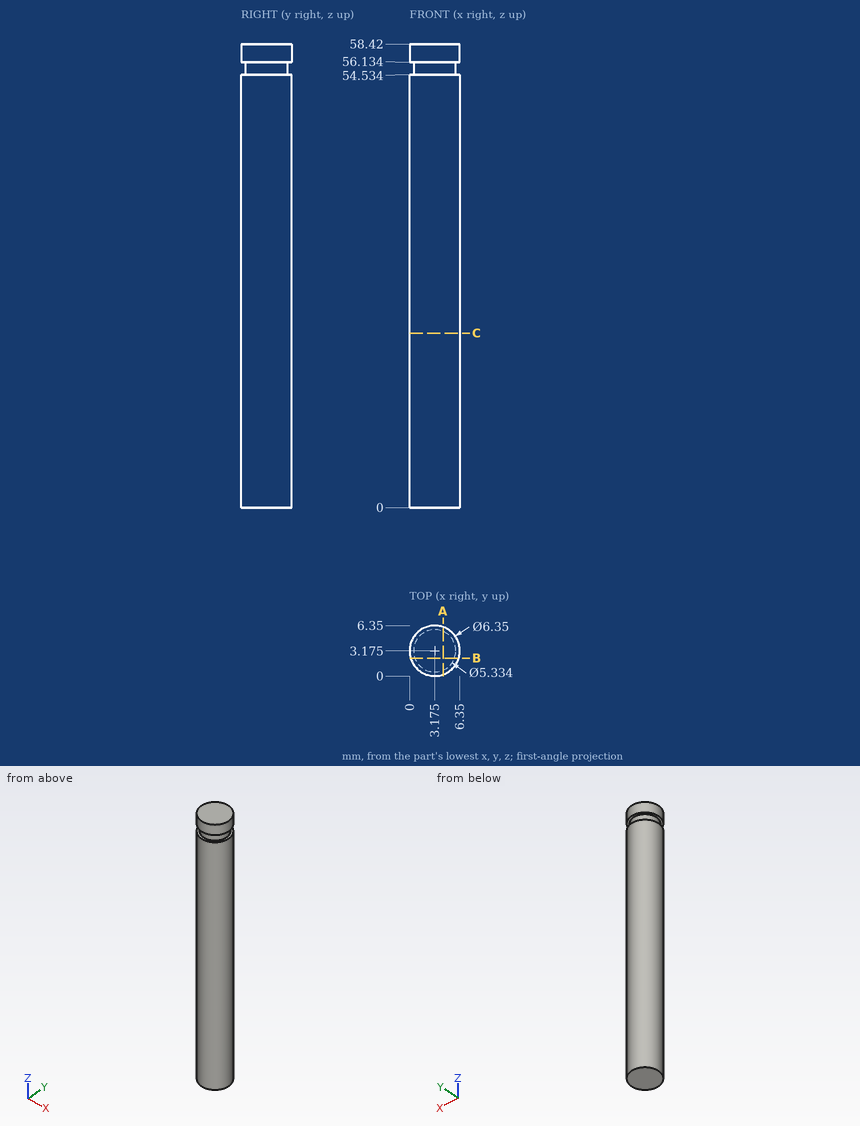
Geometry check sheet. Reference: drawing and pictorial views, mm from the part's lowest x, y, z. Give positions to 0.01 mm unless a question says otherwise; leave off trailing zeros. Write each loop counter-clockwise with the first axis right and the second up, starting at its lowest first coordinate (ties: lowest second). Pieces come first, ordered by that corner, then holes. Notation, with made-up numbers: (-8, -15.5) - (51, -15.5) arc R7 ccw to (51, -5.5) - close; hole circle Ø10 at (50.5, -14.5). An arc over 180 degrees is marked (long way). Use a Markdown table: item, result.
Q1. Section check A-A, the plane x = 4.25. Enter the section's corners in (y, z), then the cut area to 3 significant figures.
Computed:
| item | result |
|---|---|
| outline | (0.19, 0) - (6.16, 0) - (6.16, 54.53) - (5.62, 54.53) - (5.62, 56.13) - (6.16, 56.13) - (6.16, 58.42) - (0.19, 58.42) - (0.19, 56.13) - (0.73, 56.13) - (0.73, 54.53) - (0.19, 54.53) - close |
| area | 347 mm² |
Q2. Section check C-C, the plane z = 22. Enter the section's corners in (x, y) (3 decimals).
Computed:
| item | result |
|---|---|
| outline | circle Ø6.35 at (3.175, 3.175) |
Q3. Thickness scan on L1, parallel to X at y = 3, z = 16.5 (1 decimal); L2, parallel to Y at x = 3.25, z = 21; L3, parallel to X at y = 2.25, z = 22. Record the ranges inside material, lowest first. Write a range as [from, to].
Computed:
| item | result |
|---|---|
| L1 | x = [0, 6.3] |
| L2 | y = [0, 6.35] |
| L3 | x = [0.14, 6.21] |
Q4. Section check B-B, the plane y = 2.25. Enter the section's corners in (x, z), then the cut area to 3 significant figures.
Computed:
| item | result |
|---|---|
| outline | (0.14, 0) - (6.21, 0) - (6.21, 54.53) - (5.68, 54.53) - (5.68, 56.13) - (6.21, 56.13) - (6.21, 58.42) - (0.14, 58.42) - (0.14, 56.13) - (0.67, 56.13) - (0.67, 54.53) - (0.14, 54.53) - close |
| area | 353 mm² |
